from build123d import *

# Parameters (mm, degrees)
SKETCH1_R                        = 100.0125
EXTRUDE1_DEPTH                   = 6.35
SKETCH2_R                        = 93.6625
EXTRUDE2_DEPTH                   = 15.875
SKETCH3_R                        = 87.3125
CUT_EXTRUDE1_DEPTH               = 19.05
EXTRUDE3_DEPTH                   = 6.35
SKETCH5_R                        = 5.588
CUT_EXTRUDE2_DEPTH               = 153.317295267
F_10_0_1935_DIAMETER_HOLE1_D     = 4.9149
F_10_0_1935_DIAMETER_HOLE1_DEPTH = 330.2
F_10_0_1935_DIAMETER_HOLE1_TIP   = 1.476584928
FILLET1_R                        = 6.35
BOSS_EXTRUDE1_DEPTH              = 6.35
BOSS_EXTRUDE2_DEPTH              = 6.35
F_6_CLEARANCE_HOLE1_AT_2_COUNT   = 2
F_6_CLEARANCE_HOLE1_AT_2_PITCH   = 25.4


with BuildPart() as part:
    # Sketch1 → Extrude1 (new body)
    with BuildSketch(Plane.XY):
        Circle(SKETCH1_R)
    extrude(amount=EXTRUDE1_DEPTH)

    # Sketch2 → Extrude2 (add)
    with BuildSketch(Plane(origin=(0, 0, 0), x_dir=(-1, 0, 0), z_dir=(0, 0, -1))):
        with Locations(Location((0, 0, 0), (0, 0, 180))):
            Circle(SKETCH2_R)
    extrude(amount=EXTRUDE2_DEPTH)

    # Sketch3 → Cut-Extrude1 (cut)
    with BuildSketch(Plane(origin=(0, 0, -15.875), x_dir=(-1, 0, 0), z_dir=(0, 0, -1))):
        Circle(SKETCH3_R)
    extrude(amount=-CUT_EXTRUDE1_DEPTH, mode=Mode.SUBTRACT)

    # Sketch8 → Extrude3 (add)
    with BuildSketch(Plane.XY.offset(6.35)):
        with BuildLine():
            ThreePointArc((-12.674375762, 99.206150794), (0, 112.7125), (12.674375762, 99.206150794))
            ThreePointArc((12.674375762, 99.206150794), (0, 100.0125), (-12.674375762, 99.206150794))
        make_face()
        with BuildLine():
            ThreePointArc((92.25223468, -38.62674401), (97.611888324, -56.35625), (79.577858918, -60.579406784))
            ThreePointArc((79.577858918, -60.579406784), (86.613365696, -50.00625), (92.25223468, -38.62674401))
        make_face()
        with BuildLine():
            ThreePointArc((-92.25223468, -38.62674401), (-97.611888324, -56.35625), (-79.577858918, -60.579406784))
            ThreePointArc((-79.577858918, -60.579406784), (-86.613365696, -50.00625), (-92.25223468, -38.62674401))
        make_face()
    extrude(amount=-EXTRUDE3_DEPTH)

    # Sketch5 → Cut-Extrude2 (cut, through all)
    with BuildSketch(Plane.XY.offset(6.35)):
        with Locations((-63.5, -35.56)):
            Circle(SKETCH5_R)
        with Locations((63.5, -35.56)):
            Circle(SKETCH5_R)
    extrude(amount=-CUT_EXTRUDE2_DEPTH, mode=Mode.SUBTRACT)

    # #10 (0.1935) Diameter Hole1
    with Locations(Plane(origin=(0, 106.172778556, 6.35), x_dir=(1, 0, 0), z_dir=(0, 0, 1))):
        with Locations((0, 0), (91.94832342, -159.259167834), (-91.94832342, -159.259167834)):
            Hole(F_10_0_1935_DIAMETER_HOLE1_D / 2, depth=F_10_0_1935_DIAMETER_HOLE1_DEPTH)
            with Locations((0, 0, -(F_10_0_1935_DIAMETER_HOLE1_DEPTH + F_10_0_1935_DIAMETER_HOLE1_TIP / 2))):  # 118° drill point
                Cone(0, F_10_0_1935_DIAMETER_HOLE1_D / 2, F_10_0_1935_DIAMETER_HOLE1_TIP, mode=Mode.SUBTRACT)

    # Fillet1
    fillet1_edges = [part.edges().sort_by_distance(p)[0] for p in [
        (12.674375762, 99.206150794, 3.175),
        (-12.674375762, 99.206150794, 3.175),
        (79.577858918, -60.579406784, 3.175),
        (92.25223468, -38.62674401, 3.175),
        (-92.25223468, -38.62674401, 3.175),
        (-79.577858918, -60.579406784, 3.175),
    ]]
    fillet(fillet1_edges, radius=FILLET1_R)

    # Sketch25 → Boss-Extrude1 (add)
    with BuildSketch(Plane.XY.offset(6.35)):
        with BuildLine():
            ThreePointArc((-84.312132199, 53.135676765), (-86.434965165, 86.434965165), (-53.135676765, 84.312132199))
            ThreePointArc((-53.135676765, 84.312132199), (-48.681897417, 83.741957207), (-48.111722425, 88.195736555))
            ThreePointArc((-48.111722425, 88.195736555), (-90.925093226, 90.925093226), (-88.195736555, 48.111722425))
            ThreePointArc((-88.195736555, 48.111722425), (-83.741957207, 48.681897417), (-84.312132199, 53.135676765))
        make_face()
    boss_extrude1 = extrude(amount=-BOSS_EXTRUDE1_DEPTH)

    # Sketch26 → Boss-Extrude2 (add)
    with BuildSketch(Plane.XY.offset(6.35)):
        Polygon((-93.170157256, 61.739260832), (-61.739260832, 93.170157256), (-57.249132772, 88.680029196), (-88.680029196, 57.249132772), align=None)
    boss_extrude2 = extrude(amount=-BOSS_EXTRUDE2_DEPTH)

    # Sketch27 → #6 Clearance Hole1 (revolve, cut)
    with BuildSketch(Plane(origin=(-84.189901135, 66.229388893, 6.35), x_dir=(0, -1, 0), z_dir=(1, 0, 0))):
        Polygon((0, 0), (0, 26.540824014), (1.89865, 25.4), (1.89865, 0), align=None)
    f_6_clearance_hole1 = revolve(axis=Axis((-84.189901135, 66.229388893, 12.7), (0, 0, -1)), mode=Mode.SUBTRACT)

    # #6 Clearance Hole1 at 2: #6 Clearance Hole1 ×2
    with Locations(*[Vector(0.7071067811865465, 0.7071067811865487, 0) * (i * F_6_CLEARANCE_HOLE1_AT_2_PITCH) for i in range(1, F_6_CLEARANCE_HOLE1_AT_2_COUNT)]):
        add(f_6_clearance_hole1, mode=Mode.SUBTRACT)

    # Mirror1: Boss-Extrude1, Boss-Extrude2, #6 Clearance Hole1 across plane
    add(boss_extrude1.mirror(Plane(origin=(0, 0, 0), x_dir=(0, 0, 1), z_dir=(1, 0, 0))))
    add(boss_extrude2.mirror(Plane(origin=(0, 0, 0), x_dir=(0, 0, 1), z_dir=(1, 0, 0))))
    add(f_6_clearance_hole1.mirror(Plane(origin=(0, 0, 0), x_dir=(0, 0, 1), z_dir=(1, 0, 0))), mode=Mode.SUBTRACT)

    # Mirror1 copy 1 sketch → Mirror1 copy 1 (revolve, cut)
    with BuildSketch(Plane(origin=(66.229388893, 84.189901135, 6.35), x_dir=(0, -1, 0), z_dir=(-1, 0, 0))):
        Polygon((0, 0), (0, -26.540824014), (1.89865, -25.4), (1.89865, 0), align=None)
    revolve(axis=Axis((66.229388893, 84.189901135, 12.7), (0, 0, 1)), mode=Mode.SUBTRACT)


solid = part.part
Source: CAD feature listing. Evaluate the final solid. Frame: model axes, mm. A direction names the side the tool comes from. Give positions to 0.01 mm unless a question says otherwise; leave off trailing zeros. Order: outer loops, then holes, each group sorted by start corner. A loop starts at its lowest first (then second) coordinate and runs counter-clockwise, first axis right, second up. Notation, with made-up numbers: (-2.5, 84) -> (29.5, 84) arc R21 cw to (29.5, 121) -> close; hole circle Ø9 at (49, -13). An arc over 180 degrees is marked (long way). Write item = value, one per line.
Q1. Pull-direction query (X, two-part tool) for faces 5 (the face through (0.32, 108.61, 3.13)), 6 (the face through (-99.686, 8.074, 3.131)), 7 (the face through (-20.304, 91.435, -7.826)); classes: released by +X, released by -X, zero draft, split by the parting line, or undercut.
Data:
face_5 = undercut
face_6 = released by -X
face_7 = split by the parting line
Q2. Cut plane D-D, the plane x = -39.5. Output: boundary loops of the cut face in (y, z) (3 decimals), and give its area (3 significant figures).
Data:
outline = (-91.882, 0) -> (-84.926, 0) -> (-84.926, -15.875) -> (-77.867, -15.875) -> (-77.867, 3.175) -> (77.867, 3.175) -> (77.867, -15.875) -> (84.926, -15.875) -> (84.926, 0) -> (91.882, 0) -> (91.882, 6.35) -> (-91.882, 6.35) -> close
area = 897 mm^2
Q3. Cut plane B-B, the plane z = -11.5. Output: boundary loops of the cut face in (x, y) (1 decimal), and give its area (3 significant figures).
Data:
outline = circle Ø187.3 at (0, 0); hole circle Ø174.6 at (0, 0)
area = 3,610 mm^2
Q4. Cut plane C-C, the plane y = -8. Output: boundary loops of the cut face in (x, z) (3 decimals).
Data:
outline = (-99.692, 0) -> (-93.32, 0) -> (-93.32, -15.875) -> (-86.945, -15.875) -> (-86.945, 3.175) -> (86.945, 3.175) -> (86.945, -15.875) -> (93.32, -15.875) -> (93.32, 0) -> (99.692, 0) -> (99.692, 6.35) -> (-99.692, 6.35) -> close
Q5. Set-up query: faces 1 (the face through (33.254, 94.322, 3.131)), 2 (the face through (1, 1, 3.175)), 3 (the face through (77.65, 77.26, 3.22)), 4 (the face through (-1.222, -100.005, 3.131)). Return all of +Z, -Z, +X, -X, +Y, -Y with unobstructed straight access to the full face (end or side cutting, diameter ignored); none if empty.
Data:
face_1 = +Z, -Z, +Y
face_2 = -Z
face_3 = +Z, -Z
face_4 = +Z, -Z, -Y
Q6. Pin query (flat end, axial travel): pin 1 (3 mm diameter, centred on x = 16, z = -13, fed in from -Y); pin 2 (14.5 mm diameter, centred on x = -63.5, y = -35.56, fed in from -Z) (3 decimals); pin 3 (6 mm diameter, centred on x = -25.5, z = -4.5, fed in from -Y). Return the tip coordinate at first contact, or that it passes through.
Data:
pin_1 = -92.53
pin_2 = 3.175
pin_3 = -90.92
Q7. Material intervals for line 1 (Y direction, x = -63.5, z = 4); line 2 (Z direction, x = 65.5, y = 32) (3 decimals); line 3 (Y direction, x = 28.5, z = -10.5), sorted ascending. Write a range as from..to.
Data:
line_1 = -77.27..-41.15, -29.97..77.27, 82.43..91.41, 91.74..98.37
line_2 = 3.175..6.35
line_3 = -89.22..-82.53, 82.53..89.22
